CAD build for the part. Positions are in the model's coordinates, mm. Coordinates: 2 decimals unless noted, no trailing zeros. Order: outer loops, then holes, each group sorted by start corner. A loop starts at its lowest first (then second) coordinate and runs counter-clockwise, first axis right, second up.
Autodesk Inventor part; units mm, degrees
ref_plane "YZ Plane" through (0, 0, 0) normal (1, 0, 0) x (0, 1, 0)
ref_plane "XZ Plane" through (0, 0, 0) normal (0, 1, 0) x (-1, 0, 0)
ref_plane "XY Plane" through (0, 0, 0) normal (0, 0, 1) x (1, 0, 0)
sketch "Sketch1" plane through (0, 0, 0) normal (0, 0, 1) x (1, 0, 0)
  line L0 (0, 50.8) -> (-50.8, 50.8)
  line L1 (-101.6, -76.2) -> (50.8, -76.2)
  line L2 (0, 0) -> (0, 50.8) construction
  line L3 (-101.6, -76.2) -> (-101.6, -25.4)
  line L4 (-101.6, -25.4) -> (-50.8, 50.8)
  line L5 (0, 50.8) -> (50.8, -25.4)
  line L6 (50.8, -25.4) -> (50.8, -76.2)
  dimension "d0" = 50.8
  dimension "d3" = 50.8
  dimension "d17" = 127
  dimension "d18" = 50.8
  dimension "d26" = 152.4
extrude "Extrusion1" add sketch "Sketch1" along normal blind 3.175
sketch "Sketch2" plane through (0, 0, 3.175) normal (0, 0, 1) x (1, 0, 0)
  line L0 (-50.8, 50.8) -> (0, 50.8)
  line L1 (-50.8, -76.2) -> (-50.8, 50.8)
  circle A0 centre (-38.1, 38.1) radius 2.3813
  circle A1 centre (-12.7, 38.1) radius 2.3813
  circle A2 centre (-38.1, 12.7) radius 2.3813
  circle A3 centre (-12.7, 12.7) radius 2.3813
  line L2 (-38.1, 38.1) -> (-12.7, 38.1) construction
  line L3 (-12.7, 38.1) -> (-12.7, 12.7) construction
  line L4 (-12.7, 12.7) -> (-38.1, 12.7) construction
  line L5 (-38.1, 12.7) -> (-38.1, 38.1) construction
  point P0 (-101.6, -76.2)
  point P1 (0, 0)
  dimension "d6" = 4.7625
  dimension "d7" = 12.7
  dimension "d8" = 25.4
  dimension "d9" = 12.7
  dimension "d10" = 25.4
extrude "Extrusion2" cut sketch "Sketch2" against normal up to next
sketch "Sketch3" plane through (0, 0, 3.175) normal (0, 0, 1) x (1, 0, 0)
  circle A0 centre (-25.4, -25.4) radius 19.05
  point P0 (0, 0)
  dimension "d13" = 25.4
  dimension "d14" = 38.1
extrude "Extrusion3" cut sketch "Sketch3" against normal up to next
sketch "Sketch4" plane through (0, 0, 3.175) normal (0, 0, 1) x (1, 0, 0)
  circle A0 centre (-74.4647, 2.9021) radius 2.3813
  circle A1 centre (-74.4647, -54.2479) radius 2.3813
  circle A2 centre (22.9075, -25.1429) radius 2.3813
  line L0 (-74.4647, 2.9021) -> (-74.4647, -54.2479)
  point P0 (0, 0)
  dimension "d20" = 4.7625
  dimension "d23" = 57.15
extrude "Extrusion4" cut sketch "Sketch4" against normal up to next
properties part number "Plate_PictureMountPlate"
1) Drill centre lines: probe 1 along Y at (x, z) = (-38.1, 1.65); probe 2 along X at (y, z) = (37.5, 1.35); probe 3 along X at (y, z) = (-34, 0.6). Where is each one in solid material? Low to high.
2) Slice it at C-C (x = -38.1). List the corners of the cut face in (y, z) (3 decimals).
3) Two-plate mould, pull along X, no slides. Class faces 1 (the cylindrical face through (-14.455, 14.309, 1.61)), 2 (the flat face through (-26, -76.2, 2)), 3 (the flat face through (-101.6, -51, 2)): released by +X, released by -X, zero draft, split by the parting line, or undercut.
4) Slice it at D-D (z = 2). Give the number of separate pieces and of enclosed holes in the cut face, plus the area to 3 significant figures.
5) Slice it at B-B (y = -38). List the corners of the cut face in (x, z) (3 decimals).
6) Slice it at A-A (y = 12.7). List the corners of the cut face in (x, z) (3 decimals), plus the area to 3 significant figures.
Worked out:
1. probe 1: y = -76.2 to -39.6, -11.2 to 10.32, 15.08 to 35.72, 40.48 to 50.8
1. probe 2: x = -59.67 to -40.4, -35.8 to -15, -10.4 to 8.87
1. probe 3: x = -101.6 to -42.4, -8.4 to 50.8
2. outline: (-76.2, 0) - (-39.599, 0) - (-39.599, 3.175) - (-76.2, 3.175) - close; (-11.201, 0) - (10.319, 0) - (10.319, 3.175) - (-11.201, 3.175) - close; (15.081, 0) - (35.719, 0) - (35.719, 3.175) - (15.081, 3.175) - close; (40.481, 0) - (50.8, 0) - (50.8, 3.175) - (40.481, 3.175) - close
3. face 1: undercut
3. face 2: zero draft
3. face 3: released by -X
4. separate pieces: 1
4. enclosed holes: 8
4. area: 14,200 mm2
5. outline: (-101.6, 0) - (-39.688, 0) - (-39.688, 3.175) - (-101.6, 3.175) - close; (-11.112, 0) - (50.8, 0) - (50.8, 3.175) - (-11.112, 3.175) - close
6. outline: (-76.2, 0) - (-40.481, 0) - (-40.481, 3.175) - (-76.2, 3.175) - close; (-35.719, 0) - (-15.081, 0) - (-15.081, 3.175) - (-35.719, 3.175) - close; (-10.319, 0) - (25.4, 0) - (25.4, 3.175) - (-10.319, 3.175) - close
6. area: 292 mm2
